Can you work these out from the model? Positions are in its coordinate system, mm. Coordinates: 2 decimals unless noted, no trailing zeros. Order: outer loops, then holes, each group sorted by start corner. A loop starts at its lowest first (then second) coordinate and runs counter-clockwise, first axis right, second up. Notation, with made-up numbers: (64, 5.25) -> (76, 5.25) arc R15 cw to (76, 32.25) -> close; hole circle Ø3 at (71.5, 12.5). An arc over 180 degrees is marked (long way). Write item = value, one per line.
```python
from build123d import *

# Parameters (mm, degrees)
FONDO_START                   = -54
SK_FONDO_R                    = 5
FONDO_DEPTH                   = 4
PASANTES_M4_SEPARADORES_START = -54
SK_PASANTES_M4_SEPARADORES_R  = 2.25
PASANTES_M4_SEPARADORES_DEPTH = 4
AVELLANADO_M4_START           = -54
SK_AVELLANADO_M4_R            = 4.2
AVELLANADO_M4_DEPTH           = 2.5
PASANTES_M2_5_RPI_START       = -54
SK_PASANTES_M2_5_RPI_R        = 1.45
PASANTES_M2_5_RPI_DEPTH       = 4
AVELLANADO_M2_5_START         = -54
SK_AVELLANADO_M2_5_R          = 2.5
AVELLANADO_M2_5_DEPTH         = 1.5
AGUJEROS_ANCLAJE_START        = -54
SK_AGUJEROS_ANCLAJE_R         = 3.3
AGUJEROS_ANCLAJE_DEPTH        = 4
CROQUIS3_W                    = 30
CROQUIS3_H                    = 4
CROQUIS3_W_2                  = 4
CROQUIS3_H_2                  = 30
CORTAR_EXTRUIR1_DEPTH         = 177.821944339


with BuildPart() as part:
    # Sk_Fondo → Fondo (new body)
    with BuildSketch(Plane.XY.offset(FONDO_START)):
        with BuildLine():
            Line((-110, 15), (-110, 95))
            ThreePointArc((-110, 95), (-120.606601718, 120.606601718), (-95, 110))
            Line((-95, 110), (95, 110))
            ThreePointArc((95, 110), (120.606601718, 120.606601718), (110, 95))
            Line((110, 95), (110, 15))
            ThreePointArc((110, 15), (125, 0), (110, -15))
            Line((110, -15), (110, -95))
            ThreePointArc((110, -95), (120.606601718, -120.606601718), (95, -110))
            Line((95, -110), (-95, -110))
            ThreePointArc((-95, -110), (-120.606601718, -120.606601718), (-110, -95))
            Line((-110, -95), (-110, -15))
            ThreePointArc((-110, -15), (-125, 0), (-110, 15))
        make_face()
        with Locations((-110, 110)):
            Circle(SK_FONDO_R, mode=Mode.SUBTRACT)
        with Locations((110, 110)):
            Circle(SK_FONDO_R, mode=Mode.SUBTRACT)
        with Locations((110, 0)):
            Circle(SK_FONDO_R, mode=Mode.SUBTRACT)
        with Locations((110, -110)):
            Circle(SK_FONDO_R, mode=Mode.SUBTRACT)
        with Locations((-110, -110)):
            Circle(SK_FONDO_R, mode=Mode.SUBTRACT)
        with Locations((-110, 0)):
            Circle(SK_FONDO_R, mode=Mode.SUBTRACT)
    extrude(amount=FONDO_DEPTH)

    # Sk_Pasantes_M4_separadores → Pasantes_M4_separadores (cut)
    with BuildSketch(Plane.XY.offset(PASANTES_M4_SEPARADORES_START)):
        with Locations((-95, -95)):
            Circle(SK_PASANTES_M4_SEPARADORES_R)
        with Locations((-95, 95)):
            Circle(SK_PASANTES_M4_SEPARADORES_R)
        with Locations((95, -95)):
            Circle(SK_PASANTES_M4_SEPARADORES_R)
        with Locations((95, 95)):
            Circle(SK_PASANTES_M4_SEPARADORES_R)
    extrude(amount=PASANTES_M4_SEPARADORES_DEPTH, mode=Mode.SUBTRACT)

    # Sk_Avellanado_M4 → Avellanado_M4 (cut)
    with BuildSketch(Plane.XY.offset(AVELLANADO_M4_START)):
        with Locations((-95, -95)):
            Circle(SK_AVELLANADO_M4_R)
        with Locations((-95, 95)):
            Circle(SK_AVELLANADO_M4_R)
        with Locations((95, -95)):
            Circle(SK_AVELLANADO_M4_R)
        with Locations((95, 95)):
            Circle(SK_AVELLANADO_M4_R)
    extrude(amount=AVELLANADO_M4_DEPTH, mode=Mode.SUBTRACT)

    # Sk_Pasantes_M2-5_RPi → Pasantes_M2-5_RPi (cut)
    with BuildSketch(Plane.XY.offset(PASANTES_M2_5_RPI_START)):
        with Locations((-13.5, -24.5)):
            Circle(SK_PASANTES_M2_5_RPI_R)
        with Locations((-13.5, 24.5)):
            Circle(SK_PASANTES_M2_5_RPI_R)
        with Locations((-71.5, -24.5)):
            Circle(SK_PASANTES_M2_5_RPI_R)
        with Locations((-71.5, 24.5)):
            Circle(SK_PASANTES_M2_5_RPI_R)
    extrude(amount=PASANTES_M2_5_RPI_DEPTH, mode=Mode.SUBTRACT)

    # Sk_Avellanado_M2-5 → Avellanado_M2-5 (cut)
    with BuildSketch(Plane.XY.offset(AVELLANADO_M2_5_START)):
        with Locations((-13.5, -24.5)):
            Circle(SK_AVELLANADO_M2_5_R)
        with Locations((-13.5, 24.5)):
            Circle(SK_AVELLANADO_M2_5_R)
        with Locations((-71.5, -24.5)):
            Circle(SK_AVELLANADO_M2_5_R)
        with Locations((-71.5, 24.5)):
            Circle(SK_AVELLANADO_M2_5_R)
    extrude(amount=AVELLANADO_M2_5_DEPTH, mode=Mode.SUBTRACT)

    # Sk_Agujeros_anclaje → Agujeros_anclaje (cut)
    with BuildSketch(Plane.XY.offset(AGUJEROS_ANCLAJE_START)):
        with Locations((-100, -40)):
            Circle(SK_AGUJEROS_ANCLAJE_R)
        with Locations((-100, 40)):
            Circle(SK_AGUJEROS_ANCLAJE_R)
        with Locations((100, -40)):
            Circle(SK_AGUJEROS_ANCLAJE_R)
        with Locations((100, 40)):
            Circle(SK_AGUJEROS_ANCLAJE_R)
    extrude(amount=AGUJEROS_ANCLAJE_DEPTH, mode=Mode.SUBTRACT)

    # Croquis3 → Cortar-Extruir1 (cut, through all)
    with BuildSketch(Plane.XY.offset(-50)):
        with Locations((-46, -95)):
            Rectangle(CROQUIS3_W, CROQUIS3_H)
        with Locations((46, -95)):
            Rectangle(CROQUIS3_W, CROQUIS3_H)
        with Locations((46, 95)):
            Rectangle(CROQUIS3_W, CROQUIS3_H)
        with Locations((-46, 95)):
            Rectangle(CROQUIS3_W, CROQUIS3_H)
        with Locations((-93, -65.98)):
            Rectangle(CROQUIS3_W_2, CROQUIS3_H_2)
        with Locations((-93, 65.98)):
            Rectangle(CROQUIS3_W_2, CROQUIS3_H_2)
        with Locations((93, 65.98)):
            Rectangle(CROQUIS3_W_2, CROQUIS3_H_2)
        with Locations((93, -65.98)):
            Rectangle(CROQUIS3_W_2, CROQUIS3_H_2)
    extrude(amount=-CORTAR_EXTRUIR1_DEPTH, mode=Mode.SUBTRACT)


solid = part.part
```
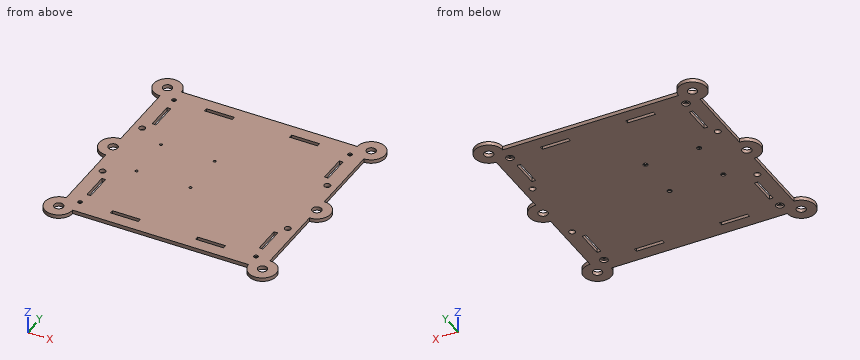
Item 1: If I drill on probe 1 along X at (y, z) = (-62.5, -50.95); probe 2 along X at (y, z) = (24.5, -51.7); probe 3 along Y at (x, z) = (-13.5, -51.6), over which ranges is the centre line in solid material (lowest first)?
A:
probe_1 = -110 to -95, -91 to 91, 95 to 110
probe_2 = -110 to -72.95, -70.05 to -14.95, -12.05 to 110
probe_3 = -110 to -25.95, -23.05 to 23.05, 25.95 to 110
Item 2: I want a section at D-D, the plane z = -53.3. Give the number of separate pieces and of enclosed holes in the cut face, plus the area to 3 significant figures.
A:
separate_pieces = 1
enclosed_holes = 26
area = 49,400 mm2
Item 3: I want a section at C-C, the plane y = 87. Please give me the cut outline in (x, z), plus the area to 3 significant figures.
A:
outline = (-110, -54) -> (110, -54) -> (110, -50) -> (-110, -50) -> close
area = 880 mm2
Item 4: I'm going to push flat-ended pins straight in: P1, Ø1, axis at x = 12, z = -52, coming from the +Y side; P2, Ø2, axis at x = -46, z = -52, coming from the -Y side; P3, Ø2, axis at y = -63.5, z = -51.5, coming from the -X side. Where does each tip first touch, or does it pass through?
A:
P1 = 110
P2 = -110
P3 = -110
Item 5: I want a section at A-A, the plane x = 56. Please give me the cut outline in (y, z).
A:
outline = (-110, -54) -> (-97, -54) -> (-97, -50) -> (-110, -50) -> close; (-93, -54) -> (93, -54) -> (93, -50) -> (-93, -50) -> close; (97, -54) -> (110, -54) -> (110, -50) -> (97, -50) -> close
Item 6: I want a section at B-B, the plane y = -40. Please give me the cut outline in (x, z).
A:
outline = (-110, -54) -> (-103.3, -54) -> (-103.3, -50) -> (-110, -50) -> close; (-96.7, -54) -> (96.7, -54) -> (96.7, -50) -> (-96.7, -50) -> close; (103.3, -54) -> (110, -54) -> (110, -50) -> (103.3, -50) -> close
